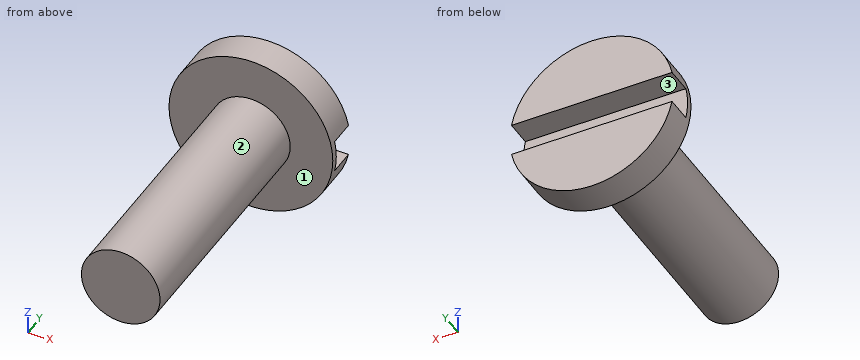
from build123d import *

# Parameters (mm, degrees)
F0_R     = 1.524
F1_DEPTH = 9.525
F2_R     = 3.175
F3_DEPTH = 1.27
F5_DEPTH = 1.016


with BuildPart() as f1:
    # F0 (on Front) → F1 (new body)
    with BuildSketch(Plane.XZ):
        Circle(F0_R)
    extrude(amount=F1_DEPTH)

    # F2 (on face) → F3 (join)
    with BuildSketch(Plane(origin=(0, 0, 0), x_dir=(-1, 0, 0), z_dir=(0, 1, 0))):
        Circle(F2_R)
    extrude(amount=F3_DEPTH)

    # F4 (on face) → F5 (cut)
    with BuildSketch(Plane(origin=(0, 1.27, 0), x_dir=(-1, 0, 0), z_dir=(0, 1, 0))):
        with BuildLine():
            ThreePointArc((3.175, 0), (3.1589222858, 0.3191159544), (3.1108519733, 0.635))
            Line((3.1108519733, 0.635), (-3.1108519733, 0.635))
            ThreePointArc((-3.1108519733, 0.635), (-3.1589222858, 0.3191159544), (-3.175, 0))
            ThreePointArc((-3.175, 0), (-3.1589222858, -0.3191159544), (-3.1108519733, -0.635))
            Line((-3.1108519733, -0.635), (3.1108519733, -0.635))
            ThreePointArc((3.1108519733, -0.635), (3.1589222858, -0.3191159544), (3.175, 0))
        make_face()
    extrude(amount=-F5_DEPTH, mode=Mode.SUBTRACT)


solid = f1.part
Here's how the part is built. I have some questions about the finished solid (model axes, mm). Face numbers are marked on the shaded views. Round coordinates to 2 decimals unless told otherwise and drop trailing zeros. Loops run counter-clockwise (first coordinate to the right, second up) from the corner with the lowest first, then second, coordinate; pieces in that order, holes last. Notation, with made-up numbers: (-24.5, 38) - (-19.5, 38) arc R34 ccw to (-19.5, 74) - close; hole circle Ø9 at (76, 81.5). An arc over 180 degrees is marked (long way). One line per question, with ' | ' between items. Start each with the question number.
Q1. We'd pull the mould along Z, two halves only. Please class the marked faces 1, 2 and 3: +Z half, -Z half, draft (parallel to the pull), parting line (faces both ways), or undercut.
Q2. I want a section at A-A (x = 0). Write out the boundary of the cut face in (y, z) (3 decimals).
Q3. Please list where these lines run through material, in increasing order: line 1 (Y direction, x = 0, z = -2.5); line 2 (Y direction, x = -1.75, z = 0.25); line 3 (X direction, y = -3.25, z = -1). Write a range as [from, to].
Q4. I want a section at C-C (y = -4.75). Write out the boundary of the cut face in (x, z), then the cut area to 3 significant figures.
Q5. I want a section at D-D (x = -1.25). Write out the boundary of the cut face in (y, z) (3 decimals).
Q6. I want a section at B-B (z = 0.5). Write out the boundary of the cut face in (x, y) (3 decimals), then the cut area to 3 significant figures.
Q7. Will this pin go through, and if not, where does the flat tip stop? pin 1 (0.5 mm diameter, centred on x = 0.5, y = 0.5, fed in from +Z).
Response values:
1) face 1: draft | face 2: parting line | face 3: undercut
2) outline: (-9.525, -1.524) - (0, -1.524) - (0, -3.175) - (1.27, -3.175) - (1.27, -0.635) - (0.254, -0.635) - (0.254, 0.635) - (1.27, 0.635) - (1.27, 3.175) - (0, 3.175) - (0, 1.524) - (-9.525, 1.524) - close
3) line 1: y = [0, 1.27] | line 2: y = [0, 0.25] | line 3: x = [-1.15, 1.15]
4) outline: circle Ø3.05 at (0, 0) | area: 7.30 mm²
5) outline: (-9.525, -0.872) - (0, -0.872) - (0, -2.919) - (1.27, -2.919) - (1.27, -0.635) - (0.254, -0.635) - (0.254, 0.635) - (1.27, 0.635) - (1.27, 2.919) - (0, 2.919) - (0, 0.872) - (-9.525, 0.872) - close
6) outline: (-3.135, 0) - (-1.44, 0) - (-1.44, -9.525) - (1.44, -9.525) - (1.44, 0) - (3.135, 0) - (3.135, 0.254) - (-3.135, 0.254) - close | area: 29.0 mm²
7) pin 1: stops at z = 3.17
